Could you check a few things on this drawing? It's one solid part, dimensions in mm from its lowest x, y, z. A direction names the side the tool comes from. Give positions to 0.01 mm unless a question says otherwise; leave off trailing zeros. Order: outer loops, then holes, each group sorted by start corner. A loop starts at its lowest first (then second) coordinate and runs counter-clockwise, first axis right, second up.
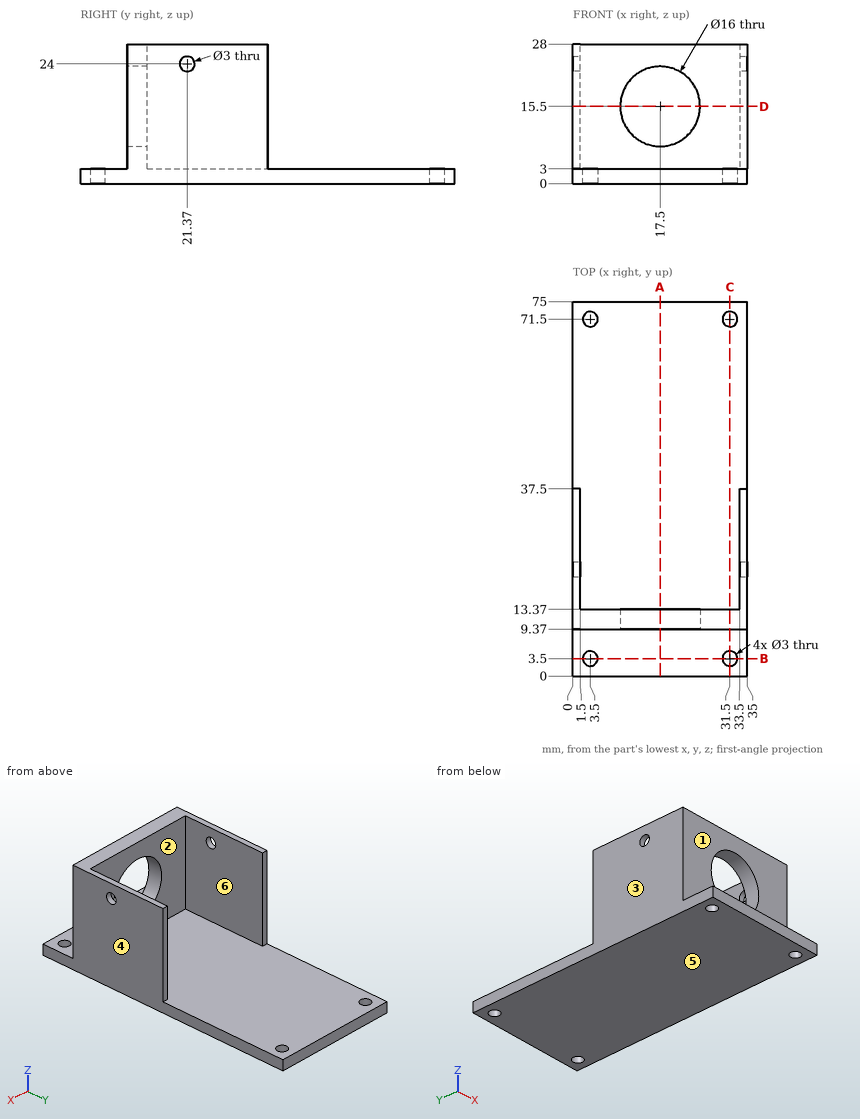
Q1. If we section it at B-B on y = 3.5: List the corners of the cut face in (x, z) for me.
Filled sheet:
outline: (0, 0) - (2, 0) - (2, 3) - (0, 3) - close; (5, 0) - (30, 0) - (30, 3) - (5, 3) - close; (33, 0) - (35, 0) - (35, 3) - (33, 3) - close
Q2. I'm going to push flat-ended pins straight in: P1, Ø1.6, axis at x = 34.5, z = 13, coming from the +Y side; P2, Ø1, axis at x = 15.5, z = 7, coming from the -Y side; P3, Ø10.5, axis at x = 23, y = 36, coming from the +Z side; P4, Ø12, axis at x = 8, y = 37.5, coming from the -Z side. Where does each tip first touch, or does it pass through?
Filled sheet:
P1: stops at y = 37.5
P2: stops at y = 9.37
P3: stops at z = 3
P4: stops at z = 0
Q3. If we section it at C-C on x = 31.5: List the corners of the cut face in (y, z) for me, plus the area to 3 significant figures.
Filled sheet:
outline: (0, 0) - (2, 0) - (2, 3) - (0, 3) - close; (5, 0) - (70, 0) - (70, 3) - (13.37, 3) - (13.37, 28) - (9.37, 28) - (9.37, 3) - (5, 3) - close; (73, 0) - (75, 0) - (75, 3) - (73, 3) - close
area: 307 mm2
Q4. I need wall thicknesses on L1, parallel to Y at x = 3.5, z = 0.75; L2, parallel to X at y = 23, z = 8.5; L3, parallel to Y at x = 34.25, z = 24. Which ranges of each line are inside material? Lowest first, please.
Filled sheet:
L1: y = 0 to 2, 5 to 70, 73 to 75
L2: x = 0 to 1.5, 33.5 to 35
L3: y = 9.37 to 19.87, 22.87 to 37.5
Q5. If we section it at D-D on z = 15.5: List the corners of the cut face in (x, y) for me, plus the area to 3 significant figures.
Filled sheet:
outline: (0, 9.37) - (9.5, 9.37) - (9.5, 13.37) - (1.5, 13.37) - (1.5, 37.5) - (0, 37.5) - close; (25.5, 9.37) - (35, 9.37) - (35, 37.5) - (33.5, 37.5) - (33.5, 13.37) - (25.5, 13.37) - close
area: 148 mm2
Q6. For the marked faces 1 and 2, which set-ups out of +Z, -Z, +X, -X, +Y, -Y let a thin tool reach every point of the face, with its end or its side?
Filled sheet:
face 1: +Z, +X, -X, -Y
face 2: +Z, +Y
Q7. Thinking about a two-plate mould opening in X: for the marked faces 3, 4, 5 and 6, which applies, released by +X, released by -X, zero draft, split by the parting line, or undercut?
Filled sheet:
face 3: released by -X
face 4: released by +X
face 5: zero draft
face 6: undercut
Q8. If we section it at A-A on x = 17.5: List the corners of the cut face in (y, z) for me, plus the area to 3 significant figures.
Filled sheet:
outline: (0, 0) - (75, 0) - (75, 3) - (13.37, 3) - (13.37, 7.5) - (9.37, 7.5) - (9.37, 3) - (0, 3) - close; (9.37, 23.5) - (13.37, 23.5) - (13.37, 28) - (9.37, 28) - close
area: 261 mm2
